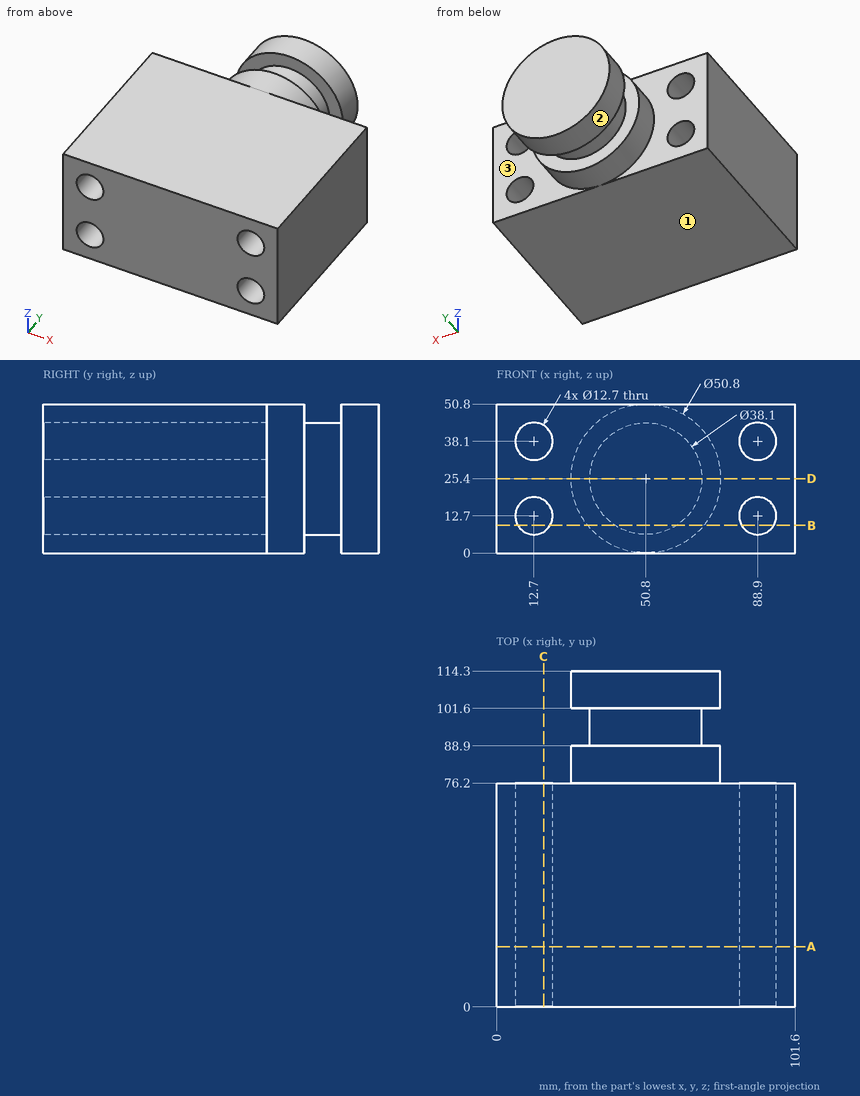
Geometry check sheet. Reference: drawing and pictorial views, mm from the part's lowest x, y, z. A direction names the side the tool comes from. Give positions to 0.01 mm unless a question says otherwise; leave off trailing zeros. Order: outer loops, then holes, each group sorted by start corner. A loop starts at its lowest first (then second) coordinate and runs counter-clockwise, first axis right, second up. Notation, with made-up numbers: (-12.75, -17.75) -> (22.25, -17.75) arc R9 cw to (22.25, -12.75) -> close; hole circle Ø6 at (81.5, 1.25). An arc over 180 degrees is marked (long way). Use CSV: the item, a comma, the result in double quotes. Start each with the question number.
1) Sectioned sample at C-C, the plane x = 16. Record the boundary of the cut face in (y, z).
2) Sectioned sample at A-A, the plane y = 20.5. Record the boundary of the cut face in (x, z).
3) Sectioned sample at B-B, the plane z = 9.5. Record the boundary of the cut face in (x, y), plus the area to 3 significant figures.
4) Sectioned sample at D-D, the plane z = 25.4. Record the boundary of the cut face in (x, y), plus the area to 3 significant figures.
5) Material ranges on line 1 (Z direction, x = 88.9, y = 49.5); line 2 (X direction, y = 56, z = 38); line 3 (X direction, y = 68.5, z = 17), recorded low to high. Write a range as from..to.
6) Go/stop test with flat-tipped pins: P1, Ø1, axis at y = 93.5, z = 31.5, coming from the +X side; P2, Ø14.5, axis at x = 12.7, z = 38.1, coming from the +Y side; P3, Ø5, axis at y = 85.5, z = 24.5, coming from the -X side. Record where each tip stops, or that it passes through.
7) Set-up check for the marked faces 1, 2 and 3: record each of +Z, -Z, +X, -X, +Y, -Y from which the full face is reachable in a straight line by a thin tool's end or side.
Recorded:
1,outline,"(0, 0) -> (76.2, 0) -> (76.2, 7.27) -> (0, 7.27) -> close; (0, 18.13) -> (76.2, 18.13) -> (76.2, 32.67) -> (0, 32.67) -> close; (0, 43.53) -> (76.2, 43.53) -> (76.2, 50.8) -> (0, 50.8) -> close"
2,outline,"(0, 0) -> (101.6, 0) -> (101.6, 50.8) -> (0, 50.8) -> close; hole circle Ø12.7 at (12.7, 12.7); hole circle Ø12.7 at (12.7, 38.1); hole circle Ø12.7 at (88.9, 12.7); hole circle Ø12.7 at (88.9, 38.1)"
3,outline,"(0, 0) -> (7.22, 0) -> (7.22, 76.2) -> (0, 76.2) -> close; (18.18, 0) -> (83.42, 0) -> (83.42, 76.2) -> (70.61, 76.2) -> (70.61, 88.9) -> (61.29, 88.9) -> (61.29, 101.6) -> (70.61, 101.6) -> (70.61, 114.3) -> (30.99, 114.3) -> (30.99, 101.6) -> (40.31, 101.6) -> (40.31, 88.9) -> (30.99, 88.9) -> (30.99, 76.2) -> (18.18, 76.2) -> close; (94.38, 0) -> (101.6, 0) -> (101.6, 76.2) -> (94.38, 76.2) -> close"
3,area,"7,340 mm2"
4,outline,"(0, 0) -> (101.6, 0) -> (101.6, 76.2) -> (76.2, 76.2) -> (76.2, 88.9) -> (69.85, 88.9) -> (69.85, 101.6) -> (76.2, 101.6) -> (76.2, 114.3) -> (25.4, 114.3) -> (25.4, 101.6) -> (31.75, 101.6) -> (31.75, 88.9) -> (25.4, 88.9) -> (25.4, 76.2) -> (0, 76.2) -> close"
4,area,"9,520 mm2"
5,line 1,"0..6.35, 19.05..31.75, 44.45..50.8"
5,line 2,"0..6.35, 19.05..82.55, 95.25..101.6"
5,line 3,"0..8.03, 17.37..84.23, 93.57..101.6"
6,P1,"x = 69.01"
6,P2,"y = 76.2"
6,P3,"x = 25.4"
7,face 1,"-Z, +X, -X, +Y, -Y"
7,face 2,"+Y"
7,face 3,"+X, +Y"
